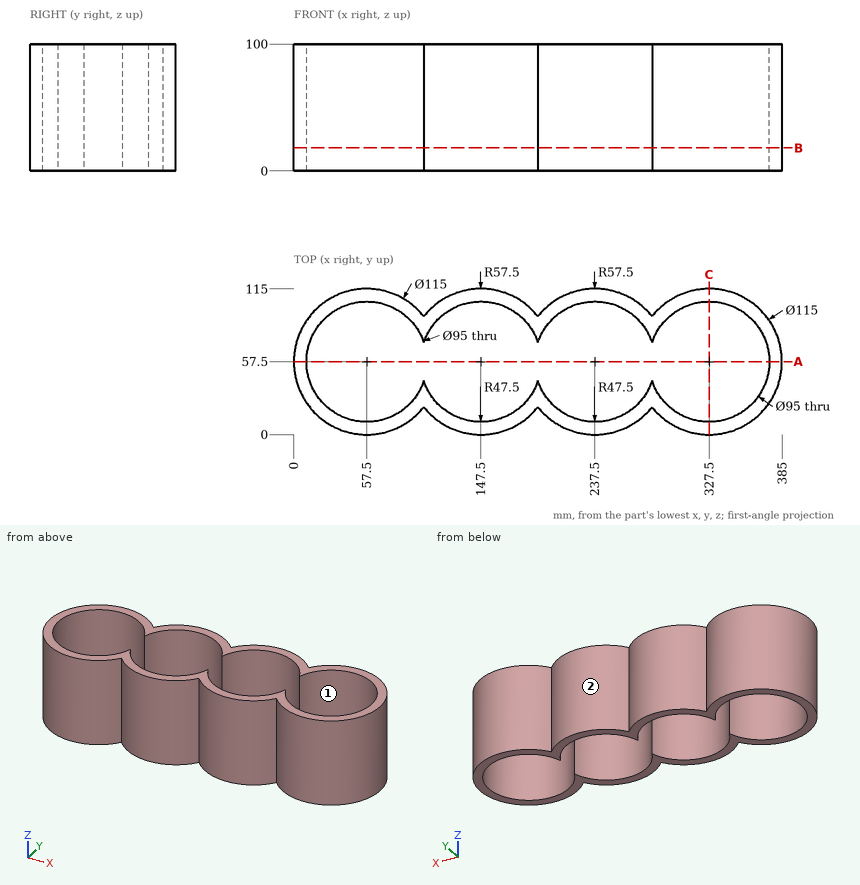
Study the drawing (mm; zero at the part's minimum x, y, z) and answer. Round coordinates to 2 decimals unless told otherwise and drop trailing zeros. Order: outer loops, then holes, each group sorted by start corner. A loop starts at its lowest first (then second) coordinate and runs counter-clockwise, first axis right, second up. Notation, with made-up numbers: (29, 44) -> (88, 44) arc R24 cw to (88, 55) -> close; hole circle Ø6 at (72, 44.25). An arc over 180 degrees is marked (long way). Answer as CSV lines item,"result". Start each with the question number.
(1) The part is cut by section C-C (x = 327.5). Determine the outline of the cut face in (y, z).
(2) The part is cut by section A-A (y = 57.5). Determine the outline of the cut face in (x, z).
(3) Flat-ended cylindrical pins translate along their axes: pin 1 Ø1 at (x, z) = (122.5, 45) entering from -Y; pin 2 Ø12 at (x, z) = (308.5, 36.5) entering from -Y; pin 3 Ø5 at (y, z) = (96, 61) entering from -X. Find the tip coordinate at first contact, or state that the pin passes through.
(4) For a pull along Y with two mould halves and no side action, classify the marked faces 1 and 2 as +Y half, -Y half, draft (parallel to the pull), parting line (faces both ways), or undercut.
(5) Find the intervals of material crossed by probe 1 along Y at (x, z) = (327, 79); probe 2 along X at (y, z) = (107.5, 90); probe 3 along X at (y, z) = (75, 60.5), in increasing order. Write a range as from..to.
(6) The part is cut by section B-B (z = 18). Determine the outline of the cut face in (x, y), then the cut area to 3 significant figures.
Evaluation:
1,outline,"(0, 0) -> (10, 0) -> (10, 100) -> (0, 100) -> close; (105, 0) -> (115, 0) -> (115, 100) -> (105, 100) -> close"
2,outline,"(0, 0) -> (10, 0) -> (10, 100) -> (0, 100) -> close; (375, 0) -> (385, 0) -> (385, 100) -> (375, 100) -> close"
3,pin 1,"y = 5.48"
3,pin 2,"y = 1.49"
3,pin 3,"x = 12.66"
4,face 1,"undercut"
4,face 2,"+Y half"
5,probe 1,"0..10, 105..115"
5,probe 2,"29.11..85.89, 119.11..175.89, 209.11..265.89, 299.11..355.89"
5,probe 3,"2.73..13.34, 101.66..103.34, 191.66..193.34, 281.66..283.34, 371.66..382.27"
6,outline,"(102.5, 21.71) arc R57.5 ccw to (192.5, 21.71) arc R57.5 ccw to (282.5, 21.71) arc R57.5 ccw (long way) to (282.5, 93.29) arc R57.5 ccw to (192.5, 93.29) arc R57.5 ccw to (102.5, 93.29) arc R57.5 ccw (long way) to start; hole (102.5, 42.29) arc R47.5 ccw to (192.5, 42.29) arc R47.5 ccw to (282.5, 42.29) arc R47.5 ccw (long way) to (282.5, 72.71) arc R47.5 ccw to (192.5, 72.71) arc R47.5 ccw to (102.5, 72.71) arc R47.5 ccw (long way) to start"
6,area,"9,840 mm²"
